from build123d import *

# Parameters (mm, degrees)
SKETCH1_R               = 5
BOSS_EXTRUDE1_DEPTH     = 60
SKETCH2_R               = 6
BOSS_EXTRUDE2_DEPTH     = 161
SKETCH3_R               = 0.5
CUT_EXTRUDE1_DEPTH      = 1.5
CUT_EXTRUDE1_DEPTH_BACK = 12.5
SKETCH4_W               = 10
SKETCH4_H               = 4.936159812
CUT_EXTRUDE2_DEPTH      = 1.5
M5_TAPPED_HOLE1_D       = 4.2
M5_TAPPED_HOLE1_DEPTH   = 10
M5_TAPPED_HOLE1_TIP     = 1.2618073
CHAMFER1_SIZE           = 3
CHAMFER2_SIZE           = 0.5
SKETCH8_W               = 5
SKETCH8_H               = 30
CUT_EXTRUDE3_DEPTH      = 161


with BuildPart() as part:
    # Sketch1 → Boss-Extrude1 (new body)
    with BuildSketch(Plane.XY):
        Circle(SKETCH1_R)
    extrude(amount=BOSS_EXTRUDE1_DEPTH)

    # Sketch2 → Boss-Extrude2 (add)
    with BuildSketch(Plane.XY.offset(60)):
        Circle(SKETCH2_R)
    extrude(amount=BOSS_EXTRUDE2_DEPTH)

    # Sketch3 → Cut-Extrude1 (cut, two sides)
    with BuildSketch(Plane(origin=(5.5, 0, 0), x_dir=(0, 0, -1), z_dir=(1, 0, 0))) as cut_extrude1_sk:
        with Locations((-36, 0)):
            Circle(SKETCH3_R)
    extrude(amount=CUT_EXTRUDE1_DEPTH, mode=Mode.SUBTRACT)
    extrude(cut_extrude1_sk.sketch, amount=-CUT_EXTRUDE1_DEPTH_BACK, mode=Mode.SUBTRACT)

    # Sketch4 → Cut-Extrude2 (cut, through all)
    with BuildSketch(Plane(origin=(5.5, 0, 0), x_dir=(0, 0, -1), z_dir=(1, 0, 0))):
        with Locations((-78.5, 0)):
            Rectangle(SKETCH4_W, SKETCH4_H)
    extrude(amount=CUT_EXTRUDE2_DEPTH, mode=Mode.SUBTRACT)

    # M5 Tapped Hole1
    with Locations(Plane(origin=(0, 0, 0), x_dir=(-1, 0, 0), z_dir=(0, 0, -1))):
        with Locations((0, 0)):
            Hole(M5_TAPPED_HOLE1_D / 2, depth=M5_TAPPED_HOLE1_DEPTH)
            with Locations((0, 0, -(M5_TAPPED_HOLE1_DEPTH + M5_TAPPED_HOLE1_TIP / 2))):  # 118° drill point
                Cone(0, M5_TAPPED_HOLE1_D / 2, M5_TAPPED_HOLE1_TIP, mode=Mode.SUBTRACT)

    # Chamfer1
    chamfer1_edges = [part.edges().sort_by_distance(p)[0] for p in [
        (-6, 0, 221),
    ]]
    chamfer(chamfer1_edges, length=CHAMFER1_SIZE)

    # Chamfer2
    chamfer2_edges = [part.edges().sort_by_distance(p)[0] for p in [
        (-5, 0, 0),
    ]]
    chamfer(chamfer2_edges, length=CHAMFER2_SIZE)

    # Sketch8 → Cut-Extrude3 (cut)
    with BuildSketch(Plane(origin=(0, -5.5, 0), x_dir=(1, 0, 0), z_dir=(0, 1, 0))):
        with Locations((-0.510877728, -80)):
            Rectangle(SKETCH8_W, SKETCH8_H)
    extrude(amount=-CUT_EXTRUDE3_DEPTH, mode=Mode.SUBTRACT)


solid = part.part
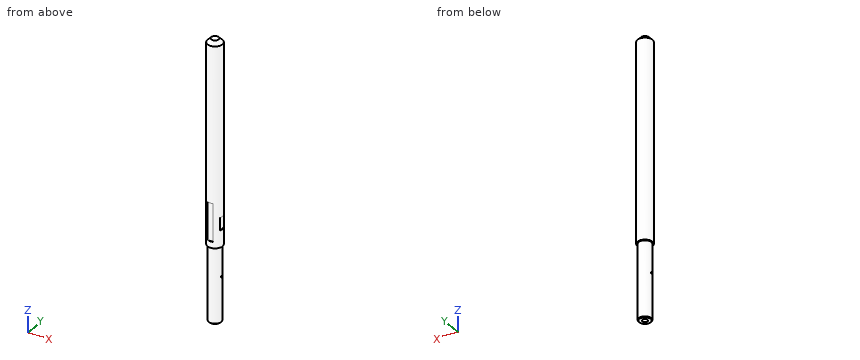
Input: part model. Units: mm. Frame: model coordinates. Give positions to 0.01 mm unless a question says otherwise; leave off trailing zeros. Write each loop counter-clockwise with the first axis right and the second up, starting at its lowest first coordinate (ties: lowest second). Pieces come first, ordered by that corner, then holes. Notation, with made-up numbers: M 45.25,68.25 L 69.25,68.25 A9 ccw 69.25,79.25 Z; hole C 16.5,27.5 d3. An arc over 180 degrees is marked long. Write item = value, one per line. Start each with the question number.
1) Cut plane A-A on z = 147. Return the cut outline in (x, y).
2) Material intervals for line 1 along Y through (x, z) = (0, 36); line 2 along Z through (x, y) = (2.25, 0); line 3 along Y through (x, z) = (-0.5, 56), sorted ascending. Write a range as [from, to].
3) First-contact query: pin 1 Ø0.6 at (x, y) = (-0.5, -6) entering from +Z; pin 2 Ø1 at (x, z) = (3.5, 75.5) entering from +Y; pin 3 Ø1 at (x, z) = (-2.5, 112.5) entering from -Y. Flat tips, straight axial feed; report the tip coordinate or a pass-through.
Solved:
q1.outline = C 0,0 d12
q2.line_1 = [-5, -0.5], [0.5, 5]
q2.line_2 = [0, 35.5], [36.5, 221]
q2.line_3 = [-4.97, 4.97]
q3.pin_1 = 218.28
q3.pin_2 = 5.2
q3.pin_3 = -5.66
